Part model, mm, in its own coordinate system. A direction names the side the tool comes from. Give positions to 0.01 mm unless a question says otherwise; leave off trailing zeros. Order: outer loops, then holes, each group sorted by start corner. A loop starts at its lowest first (then second) coordinate and runs counter-clockwise, first axis right, second up. Notation, with made-up numbers: M -35,-25 L -15,-25 A16 cw -15,-19 Z; hole C 62.5,77 d8. An arc over 180 degrees is marked long. Answer as a JSON object with one key per item and string values.
from build123d import *

# Parameters (mm, degrees)
F0_R     = 15
F1_DEPTH = 25


with BuildPart() as f1:
    # F0 (on Front) → F1 (new body)
    with BuildSketch(Plane.XZ):
        with BuildLine():
            Line((100, 150), (6.717988, 10.076982))
            ThreePointArc((6.717988, 10.076982), (1.716319, -0.51966), (0, -12.111026))
            Line((0, -12.111026), (0, -50))
            Line((0, -50), (30, -50))
            Line((30, -50), (30, -90))
            Line((30, -90), (0, -90))
            Line((0, -90), (0, -200))
            Line((0, -200), (25, -200))
            Line((25, -200), (25, -210))
            Line((25, -210), (940, -210))
            Line((940, -210), (940, -155))
            Line((940, -155), (1090, -155))
            Line((1090, -155), (1090, -40))
            ThreePointArc((1090, -40), (1078.284271, -11.715729), (1050, 0))
            Line((1050, 0), (974.188768, 0))
            ThreePointArc((974.188768, 0), (951.14683, 7.303378), (936.519091, 26.546544))
            Line((936.519091, 26.546544), (896, 140))
            Line((896, 140), (896, 0))
            Line((896, 0), (820, 0))
            Line((820, 0), (820, 140))
            Line((820, 140), (788.288901, 29.011155))
            ThreePointArc((788.288901, 29.011155), (773.915764, 8.066054), (749.827943, 0))
            Line((749.827943, 0), (729.188768, 0))
            ThreePointArc((729.188768, 0), (706.14683, 7.303378), (691.519091, 26.546544))
            Line((691.519091, 26.546544), (651, 140))
            Line((651, 140), (651, 75))
            Line((651, 75), (575, 75))
            Line((575, 75), (575, 140))
            Line((575, 140), (534.480909, 26.546544))
            ThreePointArc((534.480909, 26.546544), (519.85317, 7.303378), (496.811232, 0))
            Line((496.811232, 0), (326.40735, 0))
            ThreePointArc((326.40735, 0), (307.533033, 4.733016), (293.125339, 17.811992))
            Line((293.125339, 17.811992), (205, 150))
            Line((205, 150), (205, 0))
            Line((205, 0), (100, 0))
            Line((100, 0), (100, 150))
        make_face()
        with Locations((262, -175)):
            Circle(F0_R, mode=Mode.SUBTRACT)
        with Locations((262, -140)):
            Circle(F0_R, mode=Mode.SUBTRACT)
        with Locations((460, -175)):
            Circle(F0_R, mode=Mode.SUBTRACT)
        with Locations((460, -140)):
            Circle(F0_R, mode=Mode.SUBTRACT)
        with Locations((160, -85)):
            Circle(F0_R, mode=Mode.SUBTRACT)
        with Locations((760, -85)):
            Circle(F0_R, mode=Mode.SUBTRACT)
        with Locations((220, -30)):
            Circle(F0_R, mode=Mode.SUBTRACT)
        with Locations((262, -30)):
            Circle(F0_R, mode=Mode.SUBTRACT)
        with Locations((460, -30)):
            Circle(F0_R, mode=Mode.SUBTRACT)
        with Locations((502, -30)):
            Circle(F0_R, mode=Mode.SUBTRACT)
        with Locations((822, -30)):
            Circle(F0_R, mode=Mode.SUBTRACT)
        with Locations((902, -30)):
            Circle(F0_R, mode=Mode.SUBTRACT)
    extrude(amount=F1_DEPTH)


solid = f1.part
1. Probe line 1 along Z through (x, y) = (460, -12); line 2 along Z through (x, y) = (160, -8); line 3 along X through (y, z) = (-20.75, 38.5). List the from-to ranges inside material, lowest first.
Worked answers:
{"line 1": "z = -210 to -190, -160 to -155, -125 to -45, -15 to 0", "line 2": "z = -210 to -100, -70 to 0", "line 3": "x = 25.67 to 100, 205 to 279.33, 538.75 to 687.25, 791 to 820, 896 to 932.25"}
2. Cut at B-B on x = 160. Give the cut face in (y, z), plus the area to 3 significant figures.
Worked answers:
{"outline": "M -25,-210 L 0,-210 L 0,-100 L -25,-100 Z; M -25,-70 L 0,-70 L 0,0 L -25,0 Z", "area": "4,500 mm^2"}
3. Cut at A-A on z = -140. Give the cut face in (x, y), plus the area to 4 significant figures.
Worked answers:
{"outline": "M 0,-25 L 247,-25 L 247,0 L 0,0 Z; M 277,-25 L 445,-25 L 445,0 L 277,0 Z; M 475,-25 L 1090,-25 L 1090,0 L 475,0 Z", "area": "25,750 mm^2"}
4. Which spindle directions (+Z, -Z, +X, -X, +Y, -Y) get a long thin tool onto all of the face, cutting with end or side? Do faces 4 (the flat face through (15, -12, -50)), 5 (the flat face through (12, -12, -200)), 6 (the cylindrical face through (275.856, -12.325, -35.745)), 7 (the flat face through (1013, -12, 0)), 8 (the flat face through (651, -12, 108)). Say none if no direction does.
Worked answers:
{"face 4": "-X, +Y, -Y", "face 5": "-Z, -X, +Y, -Y", "face 6": "+Y, -Y", "face 7": "+Z, +X, +Y, -Y", "face 8": "+Z, +Y, -Y"}
5. Pin check, flat tips, straight feed: P1, Ø4, axis at y = -15.5, z = -56, coming from the -X side; P2, Ø1, axis at y = -7.5, z = 12.5, coming from the +X side; P3, Ø12.5, axis at x = 1012.5, y = -9, coming from the +Z side. Stop position of each tip, or through.
Worked answers:
{"P1": "stops at x = 30", "P2": "stops at x = 945.62", "P3": "stops at z = 0"}
6. Cut at D-D on y = -16.5. State how many separate pieces and enclosed holes the cut face has, plus the area to 3 significant figures.
Worked answers:
{"separate pieces": "1", "enclosed holes": "12", "area": "245,000 mm^2"}
7. Two-plate mould, pull along X, no slides. Class faces 1 (the flat face through (916.543, -12.325, 82.479)), 2 (the flat face through (15, -12, -90)), 3 (the flat face through (740, -12, 0)): +X half, -X half, draft (parallel to the pull), parting line (faces both ways), or undercut.
Worked answers:
{"face 1": "+X half", "face 2": "draft", "face 3": "undercut"}
8. Cut at C-C on z = -30. Give the cut face in (x, y).
Worked answers:
{"outline": "M 0,-25 L 205,-25 L 205,0 L 0,0 Z; M 235,-25 L 247,-25 L 247,0 L 235,0 Z; M 277,-25 L 445,-25 L 445,0 L 277,0 Z; M 475,-25 L 487,-25 L 487,0 L 475,0 Z; M 517,-25 L 807,-25 L 807,0 L 517,0 Z; M 837,-25 L 887,-25 L 887,0 L 837,0 Z; M 917,-25 L 1088.73,-25 L 1088.73,0 L 917,0 Z"}
